Could you check a few things on this model? Use its own coordinates, in mm. Give positions to 0.01 mm unless a question says otherwise; leave off trailing zeros. Loops run counter-clockwise (first coordinate to the right, second up) from the corner with the lowest first, then second, coordinate; pieces in that order, holes last. Notation, with made-up numbers: (-18.5, -32.75) - (7.5, -32.75) arc R32 ccw to (7.5, 6.25) - close; hole circle Ø9 at (-36, 61.25). An arc over 180 degrees is marked (long way). Write each question's results on one line, items separated by ' | '. Start each with the question number.
1) If we mould it in two halves opening along X, with no side actions, what happens to faces 1 (the face through (0.84, 38.09, 84.52)), 2 (the face through (-6, 35, 0)), 3 (the face through (1.42, 36.47, 4.53))? For each: +X half, -X half, draft (parallel to the pull), parting line (faces both ways), or undercut.
2) I want a section at B-B, the plane z = 24. Write out the boundary of the cut face in (x, y) (3 decimals).
3) If I drill on probe 1 along Z at (x, y) = (0, 35); probe 2 along X at (y, z) = (15.5, 122); probe 3 along X at (y, z) = (32, 66), over which ranges is the centre line in solid material (lowest first)? Write a range as [from, to].
4) I want a section at A-A, the plane x = 0. Write out the boundary of the cut face in (y, z) (3 decimals).
5) I want a section at C-C, the plane x = -14. Write out the boundary of the cut face in (y, z), and give its area (3 significant figures).
6) I'm going to push flat-ended pins straight in: pin 1 (2 mm diameter, centred on x = 9, z = 82, fed in from +Y); pin 2 (6 mm diameter, centred on y = 30, z = 47.5, fed in from -X); pin 3 (2 mm diameter, centred on x = 8.5, z = 17.5, fed in from -Y). Where does each tip first touch, or does it pass through?
from build123d import *

# Parameters (mm, degrees)
BOSS_EXTRUDE1_DEPTH             = 171.45
F_9_64_0_14063_DIAMETER_HOLE1_D = 3.572002


with BuildPart() as part:
    # Sketch1 → Boss-Extrude1 (new body)
    with BuildSketch(Plane.XY):
        with BuildLine():
            Line((-38.1, 0), (-34.925, 0))
            ThreePointArc((-34.925, 0), (0, 34.925), (34.925, 0))
            Line((34.925, 0), (38.1, 0))
            ThreePointArc((38.1, 0), (0, 38.1), (-38.1, 0))
        make_face()
    extrude(amount=BOSS_EXTRUDE1_DEPTH)

    # 9/64 (0.14063) Diameter Hole1 (through all)
    with Locations(Plane(origin=(0, 38.1, 0), x_dir=(1, 0, 0), z_dir=(0, 1, 0))):
        with Locations((0, -3.44678)):
            Hole(F_9_64_0_14063_DIAMETER_HOLE1_D / 2)


solid = part.part
Answers:
1) face 1: parting line | face 2: draft | face 3: undercut
2) outline: (-38.1, 0) - (-34.925, 0) arc R34.925 cw to (34.925, 0) - (38.1, 0) arc R38.1 ccw to start
3) probe 1: z = [0, 1.66], [5.23, 171.45] | probe 2: x = [-34.8, -31.3], [31.3, 34.8] | probe 3: x = [-20.68, -13.99], [13.99, 20.68]
4) outline: (34.925, 0) - (38.1, 0) - (38.1, 1.661) - (34.925, 1.661) - close; (34.925, 5.233) - (38.1, 5.233) - (38.1, 171.45) - (34.925, 171.45) - close
5) outline: (32, 0) - (35.43, 0) - (35.43, 171.45) - (32, 171.45) - close | area: 590 mm2
6) pin 1: stops at y = 37.25 | pin 2: stops at x = -26.88 | pin 3: stops at y = 33.61
